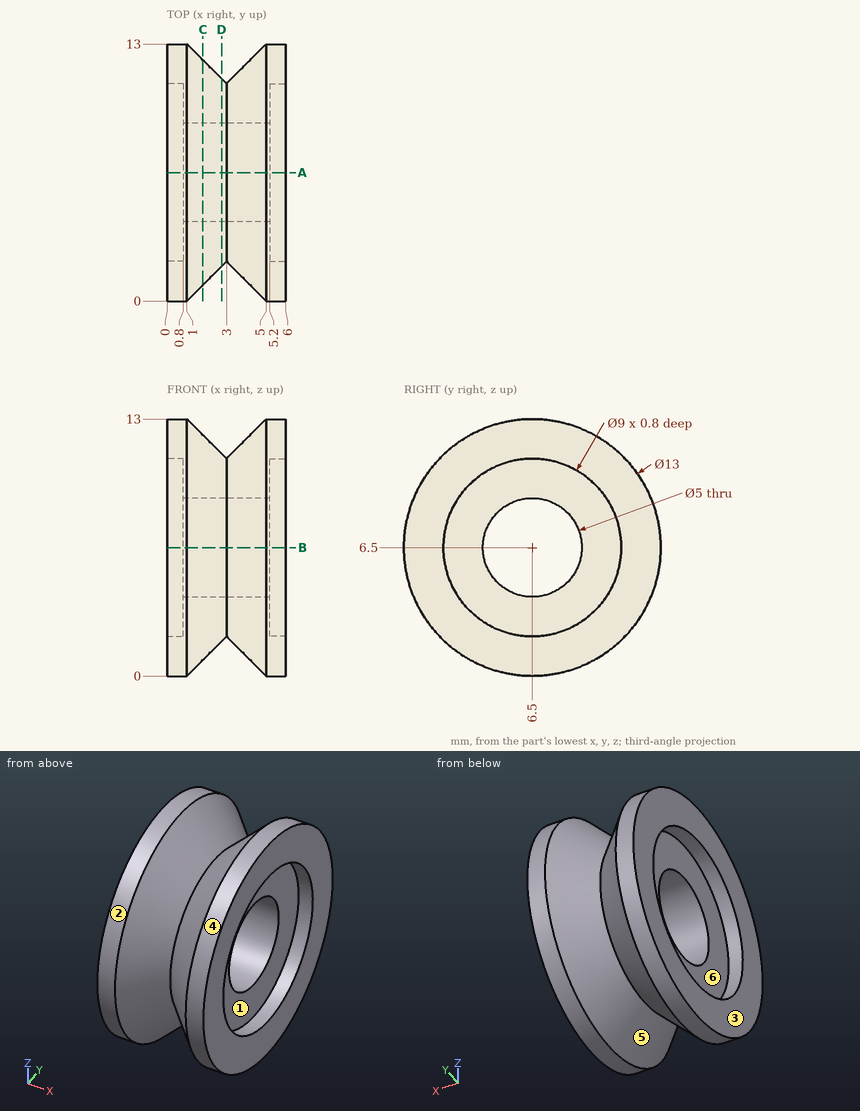
Geometry: see drawing. Coordinates: mm, zero at the bounding-box minimum. A direction names the side the tool comes from. Give positions to 0.01 mm unless a question says otherwise; leave off trailing zeros. Loops run counter-clockwise (first coordinate to the right, second up) from the corner with the lowest first, then second, coordinate; pieces in that order, holes last. Notation, with made-up numbers: (62, 57.5) -> (82, 57.5) arc R22 ccw to (82, 78.5) -> close; hole circle Ø9 at (55, 67.5). An arc over 180 degrees is marked (long way). Put each result on its own line as item: value.
1. Cut plane C-C (x = 1.8). Return the cut outline in (y, z).
Taken from the geometry:
outline: circle Ø11.4 at (6.5, 6.5); hole circle Ø5 at (6.5, 6.5)
2. Pull-direction query (Y, two-part tool) for the marked faces 1, 2 and 3; classes: released by +Y, released by -Y, zero draft, split by the parting line, or undercut.
Taken from the geometry:
face 1: undercut
face 2: split by the parting line
face 3: zero draft
3. Pin query (flat end, axial travel): P1, Ø2.5, axis at y = 7, z = 8.5, coming from the -X side; P2, Ø1, axis at x = 4.5, y = 2, coming from the -Z side; P3, Ø1.5, axis at x = 2, z = 8, coming from the +Y side. Return the tip coordinate at first contact, or that it passes through.
Taken from the geometry:
P1: stops at x = 0.8
P2: stops at z = 1.67
P3: stops at y = 12.59
4. Cut plane D-D (x = 2.75). Return the cut outline in (y, z), plus the area to 3 significant figures.
Taken from the geometry:
outline: circle Ø9.5 at (6.5, 6.5); hole circle Ø5 at (6.5, 6.5)
area: 51.2 mm2
5. Cut plane A-A (y = 6.5). Return the cut outline in (x, z).
Taken from the geometry:
outline: (0, 0) -> (1, 0) -> (3, 2) -> (5, 0) -> (6, 0) -> (6, 2) -> (5.2, 2) -> (5.2, 4) -> (0.8, 4) -> (0.8, 2) -> (0, 2) -> close; (0, 11) -> (0.8, 11) -> (0.8, 9) -> (5.2, 9) -> (5.2, 11) -> (6, 11) -> (6, 13) -> (5, 13) -> (3, 11) -> (1, 13) -> (0, 13) -> close
6. Ray query, line 1 along Y through (x, z) = (5.4, 6.5); line 2 along Z through (x, y) = (0.65, 5); line 3 along Y through (x, z) = (2.1, 6). Return the intervals inside material, ascending. Write a range as [from, to].
Taken from the geometry:
line 1: y = [0, 2], [11, 13]
line 2: z = [0.18, 2.26], [10.74, 12.82]
line 3: y = [1.12, 4.05], [8.95, 11.88]
7. Set-up query: the marked faces 4, 5 and 6. Return all of +Z, -Z, +X, -X, +Y, -Y with unobstructed straight access to the full face (end or side cutting, diameter ignored); none if empty.
Taken from the geometry:
face 4: +X, -X
face 5: none
face 6: -X
